```python
from build123d import *

# Parameters (mm, degrees)
SKETCH1_R           = 12.5
BOSS_EXTRUDE1_DEPTH = 6.35
SKETCH2_R           = 0.5
CUT_EXTRUDE1_DEPTH  = 21
SKETCH4_R           = 0.5
CUT_EXTRUDE2_DEPTH  = 258.99218142


with BuildPart() as part:
    # Sketch1 → Boss-Extrude1 (new body)
    with BuildSketch(Plane(origin=(0, 0, 0), x_dir=(1, 0, 0), z_dir=(0, 1, 0))):
        with BuildLine():
            ThreePointArc((-105.118959503, -27.088673899), (-97.681658234, -22.015485729), (-90, -17.320508076))
            Line((-90, -17.320508076), (-8.75, -158.049636191))
            ThreePointArc((-8.75, -158.049636191), (0, -190.705080757), (8.75, -158.049636191))
            Line((8.75, -158.049636191), (90, -17.320508076))
            ThreePointArc((90, -17.320508076), (97.681658234, -22.015485729), (105.118959503, -27.088673899))
            Line((105.118959503, -27.088673899), (116.798843892, -10.853517582))
            ThreePointArc((116.798843892, -10.853517582), (0, 26.794919243), (-116.798843892, -10.853517582))
            Line((-116.798843892, -10.853517582), (-105.118959503, -27.088673899))
        make_face()
        with Locations(Location((0, -173.205080757, 0), (0, 0, 270))):
            Circle(SKETCH1_R, mode=Mode.SUBTRACT)
        with BuildLine():
            Line((-10, -115.884572681), (-72.122211024, -8.285746909))
            ThreePointArc((-72.122211024, -8.285746909), (-41.722825565, 1.892622903), (-10, 6.516926799))
            Line((-10, 6.516926799), (-10, -115.884572681))
        make_face(mode=Mode.SUBTRACT)
        with BuildLine():
            Line((72.122211024, -8.285746909), (10, -115.884572681))
            Line((10, -115.884572681), (10, 6.516926799))
            ThreePointArc((10, 6.516926799), (41.722825565, 1.892622903), (72.122211024, -8.285746909))
        make_face(mode=Mode.SUBTRACT)
    extrude(amount=BOSS_EXTRUDE1_DEPTH)

    # Sketch2 → Cut-Extrude1 (cut)
    with BuildSketch(Plane(origin=(-75, 0, 43.301270189), x_dir=(0.499999999999998, 0, 0.8660254037844398), z_dir=(-0.8660254037844399, 0, 0.49999999999999806))):
        with Locations((-10, 3.175)):
            Circle(SKETCH2_R)
    cut_extrude1 = extrude(amount=-CUT_EXTRUDE1_DEPTH, mode=Mode.SUBTRACT)

    # Sketch4 → Cut-Extrude2 (cut, through all)
    with BuildSketch(Plane(origin=(-18.609768778, 0, -28.803804686), x_dir=(-0.8399421946003115, 0, 0.5426758790751738), z_dir=(-0.5426758790751737, 0, -0.8399421946003114))):
        with Locations(Location((97.99421946, 3.175, 0), (0, 0, 180))):
            Circle(SKETCH4_R)
    cut_extrude2 = extrude(amount=CUT_EXTRUDE2_DEPTH, mode=Mode.SUBTRACT)

    # Mirror1: Cut-Extrude1, Cut-Extrude2 across plane
    add(cut_extrude1.mirror(Plane(origin=(0, 0, 0), x_dir=(0, 0, 1), z_dir=(1, 0, 0))), mode=Mode.SUBTRACT)
    add(cut_extrude2.mirror(Plane(origin=(0, 0, 0), x_dir=(0, 0, 1), z_dir=(1, 0, 0))), mode=Mode.SUBTRACT)


solid = part.part
```
Model file for the job. Use its own axes, mm. A direction names the side the tool comes from. Coordinates: 2 decimals unless noted, no trailing zeros. Order: outer loops, then holes, each group sorted by start corner. A loop starts at its lowest first (then second) coordinate and runs counter-clockwise, first axis right, second up. Notation, with made-up numbers: (-14.5, 75) -> (13.5, 75) arc R21 cw to (13.5, 93) -> close; hole circle Ø11 at (-32, 35). An arc over 180 degrees is marked (long way). Answer as a JSON object with one key per item and string values. Group by question number.
1) Which spindle directions (+Z, -Z, +X, -X, +Y, -Y) get a long thin tool onto all of the face, cutting with end or side? Do faces 4 (the face through (41.496, 3.131, 61.332)), 5 (the face through (-1, 6.35, 49)), 6 (the face through (-97.788, 3.131, 22.084)). Say none if no direction does.
2) Flat gauge pins, fed straight in: pin 1 (1.5 mm diameter, centred on y = 4, z = 41, fed in from +X); pin 2 (3 mm diameter, centred on y = 4.5, z = 56, fed in from -X). Where does each tip first touch, or does it go through?
3) Cut at A-A, the plane x = 0. Write the cut outline in (y, z).
4) Pull direction X, two halves, no side cores. Call faces 1 (the face through (97.58, 3.13, 21.95)), 2 (the face through (1.746, 3.131, -26.787)), 3 (the face through (-111.04, 3.13, 18.86)): +X half, -X half, draft (parallel to the pull), parting line (faces both ways), or undercut.
5) Drill centre lines: L1, parallel to X at y = 3, z = 14; L2, parallel to X at y = 1, z = 48.5; L3, parallel to X at y = 2.5, z = 55.5. Where is each one in solid material? Low to high.
6) Cut at B-B, the plane z = 82.5. Write the cut outline in (x, y).
Check values:
{
 "1": {"face 4": "+Y, -Y", "face 5": "+Z, -Z, +X, -X, +Y", "face 6": "+Z, +Y, -Y"},
 "2": {"pin 1": "stops at x = 76.76", "pin 2": "stops at x = -68.53"},
 "3": {"outline": "(0, -26.79) -> (6.35, -26.79) -> (6.35, 160.71) -> (0, 160.71) -> close; (0, 185.71) -> (6.35, 185.71) -> (6.35, 190.71) -> (0, 190.71) -> close"},
 "4": {"face 1": "undercut", "face 2": "parting line", "face 3": "-X half"},
 "5": {"L1": "x = -114.54 to -108.18, -107.06 to -68.82, -10 to 10, 68.82 to 107.06, 108.18 to 114.54", "L2": "x = -72 to -48.9, -10 to 10, 48.9 to 72", "L3": "x = -67.96 to -44.86, -10 to 10, 44.86 to 67.96"},
 "6": {"outline": "(-52.37, 0) -> (-29.27, 0) -> (-29.27, 6.35) -> (-52.37, 6.35) -> close; (-10, 0) -> (10, 0) -> (10, 6.35) -> (-10, 6.35) -> close; (29.27, 0) -> (52.37, 0) -> (52.37, 6.35) -> (29.27, 6.35) -> close"}
}
